Study the drawing (mm; zero at the part's minimum x, y, z) and answer. A direction names the side the tool comes from. Coordinates: 2 decimals unless noted, no trailing zeros. Loops run counter-clockwise (first coordinate to the right, second up) from the corner with the lowest first, then second, coordinate; pieces in that order, holes last. Notation, with made-up numbers: (-21.75, 73) -> (19.25, 73) arc R14 ccw to (19.25, 79) -> close; hole circle Ø6 at (70, -18). An arc over 180 degrees is marked (long way). One line per question, with ' | ' between items.
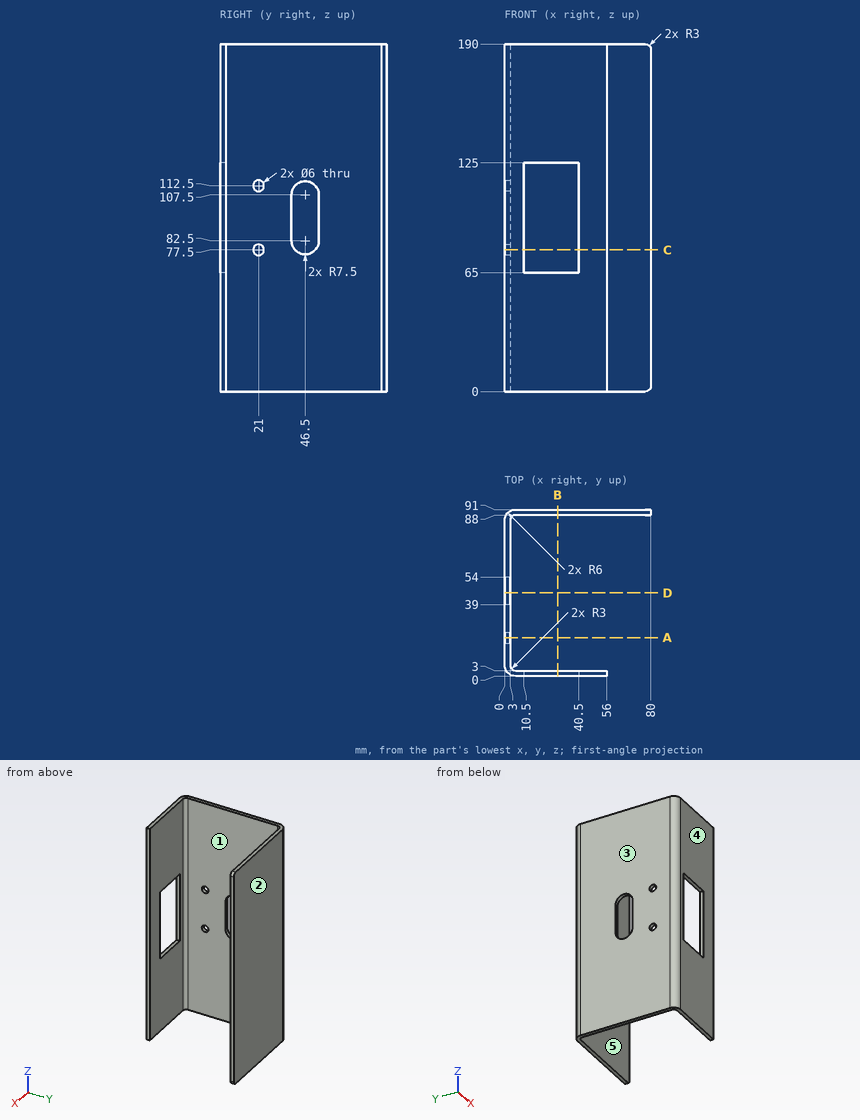
1) Find section C-C (z = 77.5). Write down the section's boundary in (x, y).
Check values:
outline: (0, 6) arc R6 ccw to (6, 0) -> (10.5, 0) -> (10.5, 3) -> (6, 3) arc R3 cw to (3, 6) -> (3, 18) -> (0, 18) -> close; (0, 24) -> (3, 24) -> (3, 40.91) -> (0, 40.91) -> close; (0, 52.09) -> (3, 52.09) -> (3, 85) arc R3 cw to (6, 88) -> (80, 88) -> (80, 91) -> (6, 91) arc R6 ccw to (0, 85) -> close; (40.5, 0) -> (56, 0) -> (56, 3) -> (40.5, 3) -> close
2) For the marked faces 4 and 5, determine the directions among +Z, -Z, +X, -X, +Y, -Y from which every point of the face is accessible in a straight line to the end or side of a thin tool.
Check values:
face 4: +Z, -Z, +X, -X, -Y | face 5: +Z, -Z, +X
3) The mould has two halves that part along Y. Classify the marked faces 1, 2 and 3: released by +Y, released by -Y, zero draft, split by the parting line, or undercut.
Check values:
face 1: undercut | face 2: released by +Y | face 3: zero draft
4) Find section D-D (y = 45.5). Write down the section's boundary in (x, z).
Check values:
outline: (0, 0) -> (3, 0) -> (3, 75.07) -> (0, 75.07) -> close; (0, 114.93) -> (3, 114.93) -> (3, 190) -> (0, 190) -> close
5) Find the intervals of material crossed by line 1 along Y through (x, z) = (54, 135.5); line 2 along Y through (x, z) = (0.9, 77.5); line 3 along Y through (x, z) = (1.2, 112.5), in increasing order.
Check values:
line 1: y = 0 to 3, 88 to 91 | line 2: y = 2.84 to 18, 24 to 40.91, 52.09 to 88.16 | line 3: y = 2.4 to 18, 24 to 40.91, 52.09 to 88.6
6) Flat-ended cylindrical pins translate along their axes: pin 1 (3.5 mm diameter, centred on y = 1.5, z = 88.5, fed in from +X); pin 2 (0.9 mm diameter, centred on x = 1.5, z = 99, fed in from +Y); pin 3 (3.5 mm diameter, centred on y = 1.5, z = 97.5, fed in from -X); pin 4 (3.5 mm diameter, centred on y = 21, z = 112.5, fed in from -X). Find the tip coordinate at first contact, or state that the pin passes through.
Check values:
pin 1: stops at x = 56 | pin 2: stops at y = 89.43 | pin 3: stops at x = 0.67 | pin 4: passes through
7) Find section A-A (y = 21). Write down the section's boundary in (x, z).
Check values:
outline: (0, 0) -> (3, 0) -> (3, 74.5) -> (0, 74.5) -> close; (0, 80.5) -> (3, 80.5) -> (3, 109.5) -> (0, 109.5) -> close; (0, 115.5) -> (3, 115.5) -> (3, 190) -> (0, 190) -> close
8) Find section B-B (x = 29). Write down the section's boundary in (y, z).
Check values:
outline: (0, 0) -> (3, 0) -> (3, 65) -> (0, 65) -> close; (0, 125) -> (3, 125) -> (3, 190) -> (0, 190) -> close; (88, 0) -> (91, 0) -> (91, 190) -> (88, 190) -> close
